For this review, take the finished solid that the model builds, in its own axes (mm). A direction names the side the tool comes from. Give positions to 0.01 mm unless a question says otherwise; leave off trailing zeros. Write each loop counter-clockwise with the first axis right and the second up, starting at its lowest first coordinate (ties: lowest second). Pieces come first, ordered by that corner, then holes.
1) We need section D-D on y = 37.75. Give the number of separate pieces and of enclosed holes in the cut face, and give its area (3 significant figures).
2) For P1, Ø10, axis at y = -28.5, z = 232, coming from the +X side; P2, Ø1.5, axis at y = 27.5, z = 198, coming from the -X side; P3, Ø5.5, axis at x = -65.38, y = -37.75, coming from the -Z side, all flat-tipped, find the tip position at first contact; note any pin that passes through.
3) We need section C-C on z = 222. Give the boundary of the cut face in (x, y), and give its area (3 significant figures).
4) We need section A-A on y = 0. Give the boundary of the cut face in (x, z), and give its area (3 significant figures).
5) Machinability: for faces 1 (the face through (5.2, 61.5, 298.123)), 2 (the face through (-61.522, 19.374, 163.486)), 3 (the face through (25.66, 66.36, 310.45)), which of the approach directions +Z, -Z, +X, -X, +Y, -Y give a long, thin tool a straight path to every point of the face, cutting with its end or side? Answer none if there is none.
6) Draft analysis for pull direction Z (two halves, no side actions). For faces 4 (the face through (57, -14, 162.5)), 5 (the face through (-0.302, 66.43, 306.414)), 6 (the face through (65.911, 23.985, 310.448)), state which applies: pulls with the +Z half, pulls with the -Z half, needs draft (parallel to the pull), parting line crosses it, or undercut.
7) Wall thickness on line 1 along Y through (x, z) = (-1, 233.5); line 2 along Y through (x, z) = (0, 163); line 3 along Y through (x, z) = (0, 171.25): over which ranges is each line inside the solid? List them lowest first.
8) We need section B-B on x = -18. Give the boundary of the cut face in (y, z), and give its area (3 significant figures).
Autodesk Inventor part; units mm, degrees
ref_plane "Work Plane1" through (0, 61.5, 0) normal (0, 1, 0) x (-1, 0, 0)
ref_plane "YZ Plane" through (0, 0, 0) normal (1, 0, 0) x (0, 1, 0)
ref_plane "XY Plane" through (0, 0, 0) normal (0, 0, 1) x (1, 0, 0)
sketch "Sketch1" plane through (0, 0, 0) normal (0, 0, 1) x (1, 0, 0)
  circle A0 centre (0, 0) radius 58.5
  circle A1 centre (0, 0) radius 61.5
  dimension "d0" = 117
  dimension "d1" = 123
extrude "Extrusion1" add sketch "Sketch1" along normal blind 323.123
ref_plane "Work Plane1" through (0, 61.5, 0) normal (0, 1, 0) x (-1, 0, 0)
sketch "Sketch2" plane through (0, 61.5, 0) normal (0, 1, 0) x (-1, 0, 0)
  line L0 (61.5, 0) -> (-61.5, 0)
  line L1 (0, 0) -> (0, 4)
  line L2 (0, 4) -> (0, 8.666)
  circle A0 centre (0, 15.524) radius 6.858
  circle A1 centre (0, 15.524) radius 7.858
  dimension "d6" = 4
  dimension "d7" = 4.666
  dimension "d8" = 13.716
  dimension "d9" = 6.858
  dimension "d33" = 15.716
extrude "Extrusion2" cut sketch "Sketch2" against normal blind 23 contours A0
thread "Thread2"
sketch "Sketch4" plane through (0, 61.5, 0) normal (0, 1, 0) x (-1, 0, 0)
  point P0 (0, 0)
sketch "Sketch5" plane through (0, 61.5, 0) normal (0, 1, 0) x (-1, 0, 0)
  line L0 (0, 0) -> (0, 76) construction
  circle A0 centre (0, 76) radius 4
  dimension "d21" = 76
  dimension "d22" = 8
extrude "Extrusion4" cut sketch "Sketch5" against normal through all
thread "Thread3"
thread "Thread4"
sketch "Sketch6" plane through (0, 0, 323.123) normal (0, 0, 1) x (1, 0, 0)
  circle A0 centre (0, 0) radius 75
  circle A1 centre (0, 0) radius 61.5
  dimension "d29" = 150
  dimension "d30" = 123
extrude "Extrusion5" add sketch "Sketch6" against normal blind 25
extrude "Extrusion6" add sketch "Sketch2" along normal blind 10
ref_plane "Work Plane2" through (0, 0, 162.5) normal (0, 0, -1) x (-1, 0, 0)
sketch "Sketch7" plane through (0, 0, 162.5) normal (0, 0, -1) x (-1, 0, 0)
  circle A0 centre (0, 0) radius 82.5
  circle A1 centre (0, 0) radius 58.5
  circle A2 centre (0, 0) radius 65.45
  circle A3 centre (0, 0) radius 75.5
  circle A4 centre (0, 75.5) radius 3
  circle A5 centre (-65.3849, 37.75) radius 3
  circle A6 centre (-65.3849, -37.75) radius 3
  circle A7 centre (0, -75.5) radius 3
  circle A8 centre (65.3849, -37.75) radius 3
  circle A9 centre (65.3849, 37.75) radius 3
  dimension "d77" = 151
  dimension "d40" = 165
  dimension "d78" = 6
  dimension "d81" = 360
split "Split3" plane through (0, 0, 162.5) removes the side toward (0, 0, -1)
sketch "Sketch8" plane through (0, 0, 323.123) normal (0, 0, 1) x (1, 0, 0)
  line L0 (0, 0) -> (0, 98.0779) construction
  line L1 (0, 0) -> (25.8311, 62.3619) construction
  circle A0 centre (25.8311, 62.3619) radius 4
  line L2 (0, 0) -> (62.3619, 25.8311) construction
  circle A1 centre (62.3619, 25.8311) radius 4
  line L3 (0, 0) -> (62.3619, -25.8311) construction
  circle A2 centre (62.3619, -25.8311) radius 4
  line L4 (0, 0) -> (25.8311, -62.3619) construction
  circle A3 centre (25.8311, -62.3619) radius 4
  line L5 (0, 0) -> (-25.8311, -62.3619) construction
  circle A4 centre (-25.8311, -62.3619) radius 4
  line L6 (0, 0) -> (-62.3619, -25.8311) construction
  circle A5 centre (-62.3619, -25.8311) radius 4
  line L7 (0, 0) -> (-62.3619, 25.8311) construction
  circle A6 centre (-62.3619, 25.8311) radius 4
  line L8 (0, 0) -> (-25.8311, 62.3619) construction
  circle A7 centre (-25.8311, 62.3619) radius 4
  dimension "d49" = 22.5
  dimension "d50" = 67.5
  dimension "d51" = 8
  dimension "d54" = 360
hole "Hole1" at (25.8311, 62.3619, 323.123) at (-25.8311, 62.3619, 323.123) at (-62.3619, 25.8311, 323.123) at (-62.3619, -25.8311, 323.123) at (62.3619, 25.8311, 323.123) at (62.3619, -25.8311, 323.123) at (25.8311, -62.3619, 323.123) at (-25.8311, -62.3619, 323.123) direction (0, 0, -1) diameter 8 depth 25
extrude "Extrusion12" add sketch "Sketch7" against normal blind 25 contours A0 | A2 | A3 A8 A7 A6 A5 A4 A9
sketch "Sketch10" plane through (0, 0, 162.5) normal (0, 0, -1) x (-1, 0, 0)
  circle A0 centre (0, 0) radius 64.5
  circle A1 centre (0, 0) radius 68
  dimension "d85" = 129
  dimension "d86" = 136
extrude "Extrusion13" cut sketch "Sketch10" against normal blind 2
ref_plane "Work Plane3" through (0, 75, 0) normal (0, 1, 0) x (-1, 0, 0)
sketch "Sketch11" plane through (0, 75, 0) normal (0, 1, 0) x (-1, 0, 0)
  line L0 (-58.5, 323.123) -> (58.5, 323.123)
  line L1 (0, 323.123) -> (0, 320.123)
  line L2 (0, 320.123) -> (0, 313.265)
  circle A0 centre (0, 313.265) radius 6.858
  point P0 (0, 0)
  dimension "d90" = 3
  dimension "d91" = 6.858
  dimension "d92" = 13.716
hole "Hole3" at (0, 75, 313.265) direction (0, -1, 0) diameter 13.716 depth 30 tip angle 118
properties part number "aluminium outer wall - front" material "Aluminum 6061"
Results list:
1. separate pieces: 4
1. enclosed holes: 0
1. area: 2,980 mm2
2. P1: stops at x = 56.83
2. P2: stops at x = -55.38
2. P3: stops at z = 298.12
3. outline: circle Ø123 at (0, 0); hole circle Ø117 at (0, 0)
3. area: 1,130 mm2
4. outline: (-82.5, 162.5) - (-68, 162.5) - (-68, 164.5) - (-64.5, 164.5) - (-64.5, 162.5) - (-58.5, 162.5) - (-58.5, 323.12) - (-75, 323.12) - (-75, 298.12) - (-61.5, 298.12) - (-61.5, 187.5) - (-82.5, 187.5) - close; (58.5, 162.5) - (64.5, 162.5) - (64.5, 164.5) - (68, 164.5) - (68, 162.5) - (82.5, 162.5) - (82.5, 187.5) - (61.5, 187.5) - (61.5, 298.12) - (75, 298.12) - (75, 323.12) - (58.5, 323.12) - close
4. area: 2,670 mm2
5. face 1: none
5. face 2: -Z
5. face 3: +Z
6. face 4: pulls with the -Z half
6. face 5: undercut
6. face 6: needs draft
7. line 1: y = -61.49 to -58.49, 58.49 to 61.49
7. line 2: y = -82.5 to -78.5, -72.5 to -68, -64.5 to -58.5, 58.5 to 64.5, 68 to 72.5, 78.5 to 82.5
7. line 3: y = -82.5 to -78.5, -72.5 to -58.5, 58.5 to 72.5, 78.5 to 82.5
8. outline: (-80.51, 162.5) - (-65.57, 162.5) - (-65.57, 164.5) - (-61.94, 164.5) - (-61.94, 162.5) - (-55.66, 162.5) - (-55.66, 323.12) - (-72.81, 323.12) - (-72.81, 298.12) - (-58.81, 298.12) - (-58.81, 187.5) - (-80.51, 187.5) - close; (55.66, 162.5) - (61.94, 162.5) - (61.94, 164.5) - (65.57, 164.5) - (65.57, 162.5) - (80.51, 162.5) - (80.51, 187.5) - (58.81, 187.5) - (58.81, 298.12) - (72.81, 298.12) - (72.81, 323.12) - (55.66, 323.12) - close
8. area: 2,780 mm2
